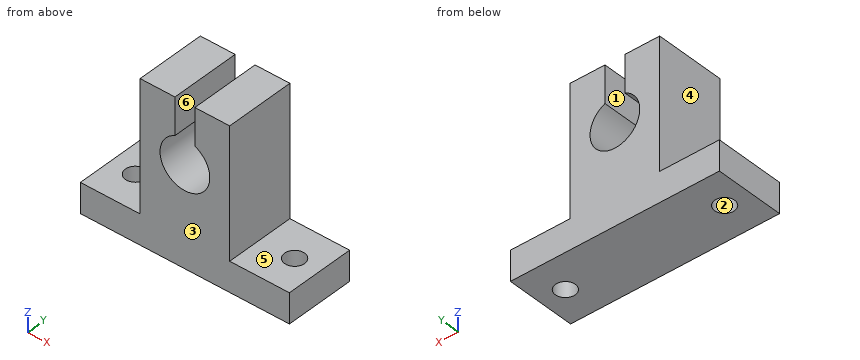
```python
from build123d import *

# Parameters (mm, degrees)
F0_W      = 42
F0_H      = 14
F1_DEPTH  = 6
F2_W      = 18
F2_H      = 14
F3_DEPTH  = 26
F4_R      = 5
F5_DEPTH  = 14
F7_W      = 4
F7_H      = 14
F8_DEPTH  = 14
F10_R     = 2
F11_DEPTH = 25


with BuildPart() as f1:
    # F0 (on Top) → F1 (new body)
    with BuildSketch(Plane.XY):
        Rectangle(F0_W, F0_H)
    extrude(amount=F1_DEPTH)

    # F2 (on face) → F3 (join)
    with BuildSketch(Plane.XY.offset(6)):
        Rectangle(F2_W, F2_H)
    extrude(amount=F3_DEPTH)

    # F4 (on face) → F5 (cut, through all)
    with BuildSketch(Plane.XZ.offset(7)):
        with Locations((0, 20)):
            Circle(F4_R)
    extrude(amount=-F5_DEPTH, mode=Mode.SUBTRACT)

    # F7 (on face) → F8 (cut)
    with BuildSketch(Plane.XY.offset(32)):
        Rectangle(F7_W, F7_H)
    extrude(amount=-F8_DEPTH, mode=Mode.SUBTRACT)

    # F10 (on face) → F11 (cut)
    with BuildSketch(Plane(origin=(0, 0, 0), x_dir=(1, 0, 0), z_dir=(0, 0, -1))):
        with Locations((16, 0)):
            Circle(F10_R)
        with Locations((-16, 0)):
            Circle(F10_R)
    extrude(amount=-F11_DEPTH, mode=Mode.SUBTRACT)


solid = f1.part
```
Geometry check sheet. Reference: the model listing, model coordinates, mm. Face numbers are marked on the shaded views. A direction names the side the tool comes from. Round coordinates to 2 decimals unless told otherwise and drop trailing zeros. Loops run counter-clockwise (first coordinate to the right, second up) from the corner with the lowest first, then second, coordinate; pieces in that order, holes last. Notation, with made-up numbers: (27.25, 11.5) - (64.25, 11.5) arc R19 ccw to (64.25, 21.5) - close; hole circle Ø6 at (-39, 14.25). An arc over 180 degrees is marked (long way). Write item = value, one per line. Start each with the question number.
1. Thickness scan on line 1 (X direction, y = 0, z = 2.3); line 2 (Y direction, x = 16, z = 2.7); line 3 (X direction, y = -2.75, z = 26). Record the ranges inside material, lowest first.
2. Set-up check for the marked faces 4, 5 and 6: record each of +Z, -Z, +X, -X, +Y, -Y from which the full face is reachable in a straight line by a thin tool's end or side.
3. Section check A-A on z = 20. Enter the section's corners in (x, y).
4. Mould release check, pull along Y, two halves, no side actions. Record for the marked faces 1, 2 and 3: released by +Y, released by -Y, zero draft, split by the parting line, or undercut.
5. Section check C-C on x = 16. Enter the section's corners in (y, z), then the cut area to 3 significant figures.
6. Section check B-B on y = 0. Enter the section's corners in (x, z).
7. Depth check by flat-ended pin: pin 1 (6 mm diameter, centred on y = 2.5, z = 27.5, fed in from -X); pin 2 (3 mm diameter, centred on x = 16, y = 0, fed in from +Z); pin 3 (6 mm diameter, centred on x = -17, y = 1.5, fed in from +Z); pin 4 (3.5 mm diameter, centred on y = -0.5, z = 28, fed in from +X). Enter the tip coordinate at first touch or a pass-through.
8. Section check D-D on z = 4. Enter the section's corners in (x, y), then the cut area to 3 significant figures.
Working result:
q1.line_1 = -21 to -18, -14 to 14, 18 to 21
q1.line_2 = -7 to -2, 2 to 7
q1.line_3 = -9 to -2, 2 to 9
q2.face_4 = +Z, -X, +Y, -Y
q2.face_5 = +Z, +X, +Y, -Y
q2.face_6 = +Z, +Y, -Y
q3.outline = (-9, -7) - (-5, -7) - (-5, 7) - (-9, 7) - close; (5, -7) - (9, -7) - (9, 7) - (5, 7) - close
q4.face_1 = zero draft
q4.face_2 = undercut
q4.face_3 = released by -Y
q5.outline = (-7, 0) - (-2, 0) - (-2, 6) - (-7, 6) - close; (2, 0) - (7, 0) - (7, 6) - (2, 6) - close
q5.area = 60.0 mm^2
q6.outline = (-21, 0) - (-18, 0) - (-18, 6) - (-21, 6) - close; (-14, 0) - (14, 0) - (14, 6) - (9, 6) - (9, 32) - (2, 32) - (2, 24.58) arc R5 cw (long way) to (-2, 24.58) - (-2, 32) - (-9, 32) - (-9, 6) - (-14, 6) - close; (18, 0) - (21, 0) - (21, 6) - (18, 6) - close
q7.pin_1 = -9
q7.pin_2 = through
q7.pin_3 = 6
q7.pin_4 = 9
q8.outline = (-21, -7) - (21, -7) - (21, 7) - (-21, 7) - close; hole circle Ø4 at (-16, 0); hole circle Ø4 at (16, 0)
q8.area = 563 mm^2
